Autodesk Fusion 360 part; units mm, degrees
sketch "Sketch1" plane through (0, 0, 0) normal (0, 1, 0) x (1, 0, 0)
  line L0 (0, 0) -> (10, 0)
  line L1 (10, 0) -> (10, -17)
  line L2 (0, -17) -> (0, 0)
  line L3 (0, -17) -> (5, -22)
  line L4 (5, -22) -> (10, -17)
  dimension "d1" = 10
  dimension "d2" = 17
extrude "Extrude1" add sketch "Sketch1" along normal blind 10
sketch "Sketch2" plane through (0, 0, 0) normal (0, 1, 0) x (1, 0, 0)
  line L0 (1, -1) -> (9, -1)
  line L1 (9, -1) -> (9, -16)
  line L2 (9, -16) -> (1, -16)
  line L3 (1, -16) -> (1, -1)
  line L4 (2, -18) -> (8, -18)
  line L5 (8, -18) -> (5, -21)
  line L6 (5, -21) -> (2, -18)
extrude "Extrude2" cut sketch "Sketch2" along normal blind 2 contours L4 L5 L6
extrude "Extrude3" cut sketch "Sketch2" along normal blind 9 contours L0 L1 L2 L3
sketch "Sketch3" plane through (0, 9, 0) normal (0, -1, 0) x (1, 0, 0)
  line L0 (9, 16) -> (1, 16)
  line L1 (1, 16) -> (1, 1)
  line L2 (1, 1) -> (9, 1)
  line L3 (9, 1) -> (9, 16)
  line L4 (1, 1) -> (9, 1)
  line L5 (9, 1) -> (9, 6.5)
  line L6 (9, 6.5) -> (1, 6.5)
  line L7 (1, 6.5) -> (1, 1)
extrude "Extrude4" add sketch "Sketch3" along normal blind 6 contours L1 L2 L3 L4 L5 L6 L7
sketch "Sketch4" plane through (0, 0, 6.5) normal (0, 0, 1) x (-1, 0, 0)
  line L0 (-9, -9) -> (-1, -9)
  line L1 (-1, -9) -> (-1, -3)
  line L2 (-1, -3) -> (-9, -3)
  line L3 (-9, -3) -> (-9, -9)
  circle A0 centre (-5, -6) radius 2.5
  circle A1 centre (-5, -6) radius 1.75
  dimension "d11" = 5
  dimension "d12" = 3.5
extrude "Extrude5" add sketch "Sketch4" along normal blind 0.5 contours A0
extrude "Extrude6" cut sketch "Sketch4" against normal blind 3 contours A1
Can you work these out from the model? Positions are in its coordinate system, mm. A direction names the side the tool comes from. Round coordinates to 2 decimals unless told otherwise and drop trailing zeros. Write each loop counter-clockwise with the first axis right and the second up, starting at its lowest first coordinate (ties: lowest second). Pieces come first, ordered by that corner, then holes. Notation, with made-up numbers: M -2.5,21 L 23.5,21 A28 cw 23.5,42 Z; hole C 84,78.25 d2. An arc over 180 degrees is marked long. Use a Markdown table: item, result.
Item 1: If I drill on line 1 along X through (y, z) = (8.5, 7); line 2 along Y through (x, z) = (5, 4.6); line 3 along Z through (x, y) = (4, 8.25), over which ranges is the centre line in solid material (lowest first)? Write a range as [from, to].
Found:
| item | result |
|---|---|
| line 1 | x = [0, 1], [9, 10] |
| line 2 | y = [3, 4.25], [7.75, 10] |
| line 3 | z = [0, 7], [16, 21] |
Item 2: I want a section at D-D (z = 3). List the corners of the cut face in (x, y) for me.
Found:
| item | result |
|---|---|
| outline | M 0,0 L 1,0 L 1,3 L 9,3 L 9,0 L 10,0 L 10,10 L 0,10 Z |
Item 3: I want a section at C-C (x = 1.75). List the corners of the cut face in (y, z) for me.
Found:
| item | result |
|---|---|
| outline | M 0,0 L 10,0 L 10,18.75 L 0,18.75 L 0,16 L 9,16 L 9,6.5 L 3,6.5 L 3,1 L 0,1 Z |
Item 4: We'd pull the mould along Y, two halves only. Please class faces 1 (the face through (5, 6, 3.5)), 2 (the face through (10, 5, 8)), 3 (the face through (5, 3, 4)): released by +Y, released by -Y, zero draft, split by the parting line, or undercut.
Found:
| item | result |
|---|---|
| face 1 | undercut |
| face 2 | zero draft |
| face 3 | released by -Y |
Item 5: I want a section at B-B (y = 6). List the corners of the cut face in (x, z) for me.
Found:
| item | result |
|---|---|
| outline | M 0,0 L 10,0 L 10,17 L 5,22 L 0,17 Z; hole M 1,6.5 L 2.5,6.5 L 2.5,7 L 3.25,7 L 3.25,3.5 L 6.75,3.5 L 6.75,7 L 7.5,7 L 7.5,6.5 L 9,6.5 L 9,16 L 1,16 Z |
Item 6: For pin 1 Ø3 at (x, y) = (5.5, 6.5) entering from +Z; pin 2 Ø0.9 at (x, y) = (7, 2) entering from +Z; pin 3 Ø6 at (x, z) = (5.5, 5) entering from -Y, each with a flat end and sliding along its axis, tell me the tip position at first contact or that it passes through.
Found:
| item | result |
|---|---|
| pin 1 | stops at z = 22 |
| pin 2 | stops at z = 20.45 |
| pin 3 | stops at y = 3 |
Item 7: I want a section at A-A (z = 12). List the corners of the cut face in (x, y) for me, and give its area (3 significant figures).
Found:
| item | result |
|---|---|
| outline | M 0,0 L 1,0 L 1,9 L 9,9 L 9,0 L 10,0 L 10,10 L 0,10 Z |
| area | 28.0 mm2 |
Item 8: Which directions (+Z, -Z, +X, -X, +Y, -Y) give clear straight access to the entire face, cutting with the end or side of a thin tool? Please do faces 4 (the face through (2, 5, 19)), 5 (the face through (9, 4, 10)), 6 (the face through (2.615, 6.751, 6.746)).
Found:
| item | result |
|---|---|
| face 4 | +Z, -X, +Y, -Y |
| face 5 | -Y |
| face 6 | none |
